Geometry: see drawing. Coordinates: mm, zero at the bounding-box minimum. Round coordinates to 2 decimals unless told otherwise and drop trailing zeros. Loops run counter-clockwise (first coordinate to the right, second up) from the corner with the lowest first, then second, coordinate; pieces in that order, holes last. Notation, with made-up numbers: (-12.5, 25.5) -> (-1.5, 25.5) arc R4 cw to (-1.5, 30.5) -> close; hole circle Ø1 at (45.5, 36.25). An arc over 180 degrees is marked (long way). Write item = value, one per line.
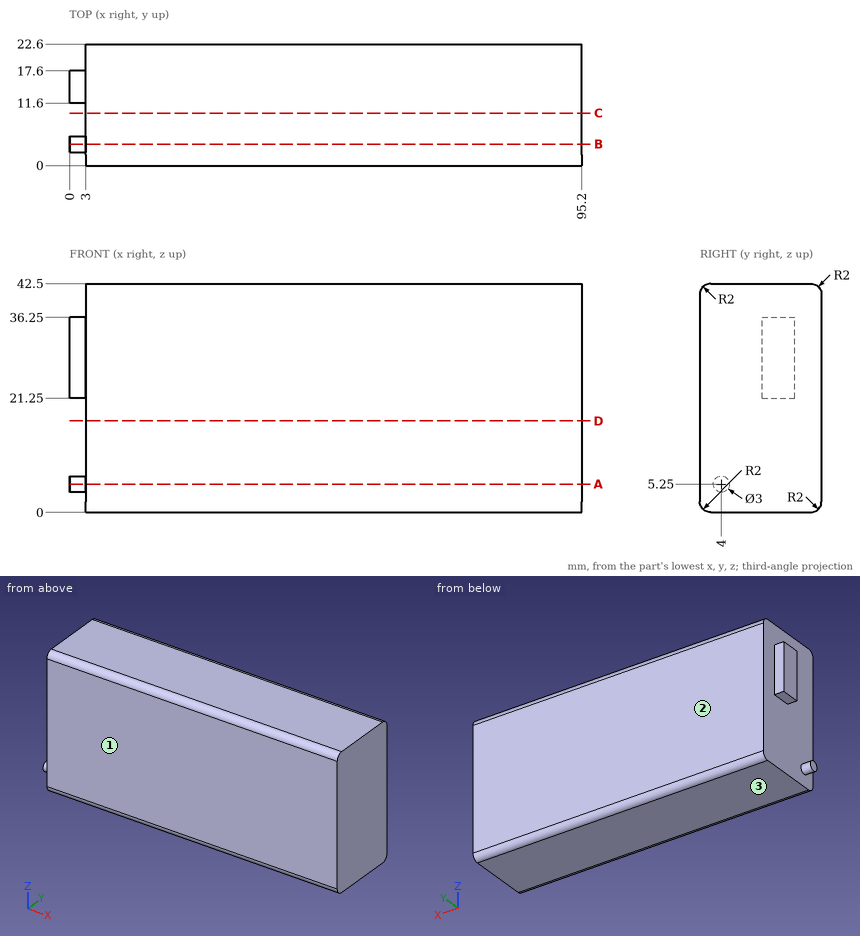
1. Section query A-A (z = 5.25). Return the cut outline in (x, y).
Evaluation:
outline = (0, 2.5) -> (3, 2.5) -> (3, 0) -> (95.2, 0) -> (95.2, 22.6) -> (3, 22.6) -> (3, 5.5) -> (0, 5.5) -> close
2. Contact query for flat-ended pins moving along their axis: pin 1 Ø4 at (y, z) = (15, 12.5) entering from -X; pin 2 Ø2.5 at (x, z) = (1, 26) entering from -Y; pin 3 Ø0.9 at (x, y) = (1.5, 16) entering from -Z. Output: stop coordinate, or through.
Evaluation:
pin_1 = 3
pin_2 = 11.6
pin_3 = 21.25
3. Line query: probe 1 along X at (y, z) = (2, 18); probe 2 along Z at (x, y) = (41.5, 1.5). Output: solid intervals per line, ascending. Write a range as from..to.
Evaluation:
probe_1 = 3..95.2
probe_2 = 0.06..42.44
4. Mould query, pull axis Y, two halves, no side actions, for the marked faces 1, 2 and 3. Classes: released by +Y, released by -Y, zero draft, split by the parting line, or undercut.
Evaluation:
face_1 = released by -Y
face_2 = released by +Y
face_3 = zero draft
5. Section query D-D (z = 17). Return the cut outline in (x, y), then the cut area to 3 significant figures.
Evaluation:
outline = (3, 0) -> (95.2, 0) -> (95.2, 22.6) -> (3, 22.6) -> close
area = 2,080 mm²
6. Section query C-C (y = 9.75). Return the cut outline in (x, z).
Evaluation:
outline = (3, 0) -> (95.2, 0) -> (95.2, 42.5) -> (3, 42.5) -> close
7. Section query B-B (y = 4). Return the cut outline in (x, z).
Evaluation:
outline = (0, 3.75) -> (3, 3.75) -> (3, 0) -> (95.2, 0) -> (95.2, 42.5) -> (3, 42.5) -> (3, 6.75) -> (0, 6.75) -> close
